Read the model definition and answer for the solid it produces. Units are mm, in the model's axes. Face numbers are marked on the shaded views. A direction names the side the tool comes from. Give positions to 0.01 mm unless a question says otherwise; leave off trailing zeros. Order: outer loops, then holes, each group sorted by start corner. A loop starts at its lowest first (then second) coordinate and runs counter-clockwise, first axis right, second up. Notation, with made-up numbers: (-19.5, 56) - (-8.5, 56) arc R25 cw to (-8.5, 69) - close; hole circle Ø2 at (50, -14.5). An arc over 180 degrees is marked (long way). Write item = value, one per line.
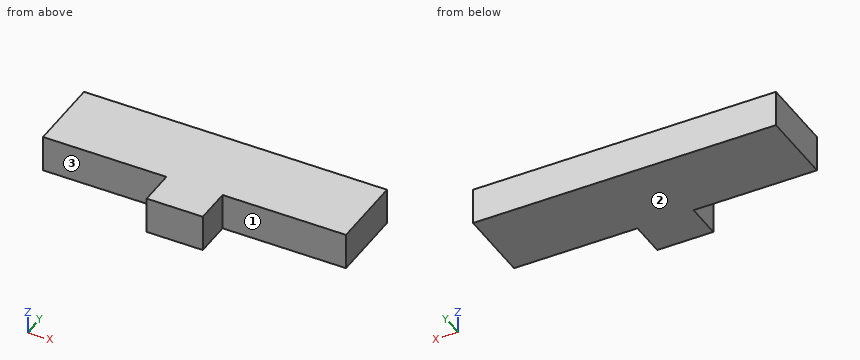
Autodesk Inventor part; units mm, degrees
ref_plane "YZ Plane" through (0, 0, 0) normal (1, 0, 0) x (0, 1, 0)
ref_plane "XZ Plane" through (0, 0, 0) normal (0, 1, 0) x (-1, 0, 0)
ref_plane "XY Plane" through (0, 0, 0) normal (0, 0, 1) x (1, 0, 0)
sketch "Block1" plane through (0, 0, 0) normal (0, 0, 1) x (1, 0, 0)
  circle A0 centre (74.029, 24.2723) radius 1
  line L0 (49.279, 30.4723) -> (71.779, 30.4723)
  line L1 (71.779, 30.4723) -> (71.779, 18.0723)
  line L2 (71.779, 18.0723) -> (49.279, 18.0723)
  line L3 (49.279, 18.0723) -> (49.279, 30.4723)
  line L4 (49.279, 30.4723) -> (44.779, 30.4723)
  line L5 (44.779, 30.4723) -> (44.779, 18.0723)
  line L6 (44.779, 18.0723) -> (49.279, 18.0723)
  line L7 (49.279, 18.0723) -> (49.279, 30.4723)
  line L8 (71.779, 30.4723) -> (76.279, 30.4723)
  line L9 (76.279, 30.4723) -> (76.279, 18.0723)
  line L10 (76.279, 18.0723) -> (71.779, 18.0723)
  line L11 (71.779, 18.0723) -> (71.779, 30.4723)
  line L12 (44.779, 24.2723) -> (76.279, 24.2723) construction
  line L13 (47.029, 30.4723) -> (47.029, 18.0723) construction
  circle A1 centre (47.029, 24.2723) radius 1
  line L14 (74.029, 30.4723) -> (74.029, 18.0723) construction
  point P0 (60.979, 24.0984)
  dimension "d7" = 22.5
  dimension "d8" = 12.4
  dimension "d9" = 4.5
  dimension "d10" = 4.5
  dimension "d11" = 2
  dimension "d12" = 2
sketch "Sketch1" plane through (0, 0, 0) normal (0, 0, 1) x (1, 0, 0)
  line L0 (-92.7646, -8.503) -> (-89.7646, -8.503)
  line L1 (-89.7646, -8.503) -> (-89.7646, -11.753)
  line L2 (-89.7646, -11.753) -> (-92.7646, -11.753)
  line L3 (-92.7646, -11.753) -> (-92.7646, -8.503)
  line L4 (-92.7646, -21.6527) -> (-89.7646, -21.6527)
  line L5 (-89.7646, -21.6527) -> (-89.7646, -21.7527)
  line L6 (-89.7646, -21.7527) -> (-92.7646, -21.7527)
  line L7 (-92.7646, -21.7527) -> (-92.7646, -21.6527)
  line L8 (8.196, 15.0005) -> (35.196, 15.0005)
  line L9 (35.196, 15.0005) -> (35.196, 8.2505)
  line L10 (35.196, 8.2505) -> (8.196, 8.2505)
  line L11 (8.196, 8.2505) -> (8.196, 15.0005)
  line L12 (8.196, 11.6255) -> (35.196, 11.6255) construction
  line L13 (21.696, 15.0005) -> (21.696, 8.2505) construction
  line L14 (19.196, 5.0005) -> (24.196, 5.0005)
  line L15 (24.196, 5.0005) -> (24.196, 8.2505)
  line L16 (24.196, 8.2505) -> (19.196, 8.2505)
  line L17 (19.196, 8.2505) -> (19.196, 5.0005)
  line L18 (21.696, 8.2505) -> (21.696, 5.0005) construction
  point P0 (0, 0)
  dimension "d0" = 3
  dimension "mat" = 3.25
  dimension "d2" = 3
  dimension "d3" = 0.1
  dimension "d59" = 27
  dimension "d60" = 6.75
  dimension "d61" = 5
  dimension "d62" = 3.25
extrude "Extrusion6" add sketch "Sketch1" along normal blind 3.25 contours L8 L9 L10 L11 | L10 L15 L14 L17
equation "\"d62\" = mat"
equation "\"d65\" = mat"
properties part number "arm-servo"
1. For the marked faces 1, 2 and 3, determine the directions among +Z, -Z, +X, -X, +Y, -Y from which every point of the face is accessible in a straight line to the end or side of a thin tool.
Recorded:
face_1 = +Z, -Z, +X, -Y
face_2 = -Z, +X, -X, +Y, -Y
face_3 = +Z, -Z, -X, -Y
2. Section C-C (y = 5.5) is taken. Determine the outline of the cut face in (x, z), and give its area (4 significant figures).
Recorded:
outline = (19.2, 0) - (24.2, 0) - (24.2, 3.25) - (19.2, 3.25) - close
area = 16.25 mm^2
3. Section A-A (z = 2.85) is taken. Determine the outline of the cut face in (x, y).
Recorded:
outline = (8.2, 8.25) - (19.2, 8.25) - (19.2, 5) - (24.2, 5) - (24.2, 8.25) - (35.2, 8.25) - (35.2, 15) - (8.2, 15) - close
4. Straight lines are drawn through the part: L1, parallel to Y at x = 14.5, z = 2.85; L2, parallel to X at y = 6.5, z = 0.15. For each, find the intervals that lie inside material, in ascending order. Write a range as [from, to].
Recorded:
L1 = [8.25, 15]
L2 = [19.2, 24.2]
5. Flat-ended cylindrical pins translate along their axes: pin 1 (1.6 mm diameter, centred on x = 28.5, z = 1, fed in from -Y); pin 2 (1 mm diameter, centred on x = 29, y = 8.5, fed in from -Z). Find the tip coordinate at first contact, or state that the pin passes through.
Recorded:
pin_1 = 8.25
pin_2 = 0
6. Section B-B (x = 30) is taken. Determine the outline of the cut face in (y, z), and give its area (3 significant figures).
Recorded:
outline = (8.25, 0) - (15, 0) - (15, 3.25) - (8.25, 3.25) - close
area = 21.9 mm^2
